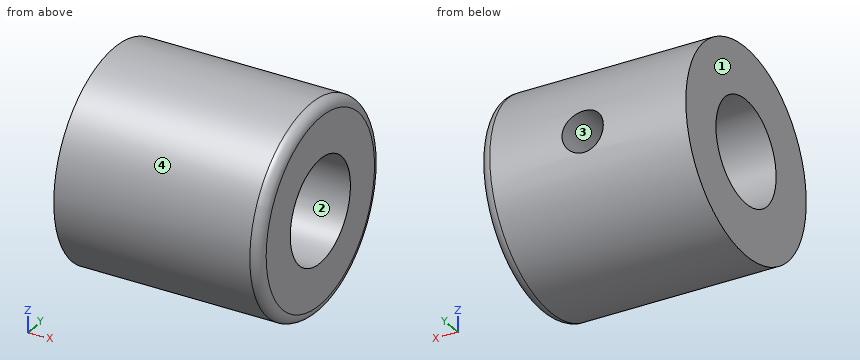
Autodesk Inventor part; units mm, degrees
ref_plane "YZ Plane" through (0, 0, 0) normal (1, 0, 0) x (0, 1, 0)
ref_plane "XZ Plane" through (0, 0, 0) normal (0, 1, 0) x (-1, 0, 0)
ref_plane "XY Plane" through (0, 0, 0) normal (0, 0, 1) x (1, 0, 0)
sketch "Sketch1" plane through (0, 0, 0) normal (1, 0, 0) x (0, 1, 0)
  circle A0 centre (0, 0) radius 2.5
  circle A1 centre (0, 0) radius 5
  dimension "d0" = 5
  dimension "d1" = 10
extrude "Extrusion1" add sketch "Sketch1" along normal blind 10
sketch "Sketch2" plane through (0, 0, 0) normal (0, 1, 0) x (-1, 0, 0)
  line L0 (0, 0) -> (-5, 0)
  circle A0 centre (-5, 0) radius 1
  dimension "d4" = 5
  dimension "d5" = 2
extrude "Extrusion2" cut sketch "Sketch2" along normal blind 10
thread "Thread1"
fillet "Fillet1" radius 0.5 1 edges at (10, -5, 0)
properties part number "wormgear_worm_axes_holder" material "Aluminum 6061"
Model file for the job. Use its own axes, mm. Face numbers are marked on the shaded views. Give positions to 0.01 mm unless a question says otherwise; leave off trailing zeros. Loops run counter-clockwise (first coordinate to the right, second up) from the corner with the lowest first, then second, coordinate; pieces in that order, holes last.
Item 1: Slice it at B-B (z = 0). Write the cut outline in (x, y), plus the area to 3 significant figures.
Check values:
outline: (0, -5) - (9.5, -5) arc R0.5 ccw to (10, -4.5) - (10, -2.5) - (0, -2.5) - close; (0, 2.5) - (4, 2.5) - (4, 5) - (0, 5) - close; (6, 2.5) - (10, 2.5) - (10, 4.5) arc R0.5 ccw to (9.5, 5) - (6, 5) - close
area: 44.9 mm2
Item 2: Slice it at C-C (x = 7.25). Write the cut outline in (y, z), plus the area to 3 significant figures.
Check values:
outline: circle Ø10 at (0, 0); hole circle Ø5 at (0, 0)
area: 58.9 mm2
Item 3: Mould opens along Z. For the marked faces 1, 2, 3 and 4 say: +Z half, -Z half, draft (parallel to the pull), parting line (faces both ways), or undercut.
Check values:
face 1: draft
face 2: undercut
face 3: undercut
face 4: parting line
Item 4: Drop a flat-ended pin along its axis: P1, Ø1.5, axis at x = 4, z = 1, coming from the +Y side. Give the stop position or say it passes through.
Check values:
P1: stops at y = 4.99
Item 5: Drill centre lines: line 1 along X through (y, z) = (2.9, 0); line 2 along Z through (x, y) = (4, 0); line 3 along Z through (x, y) = (5, 4.05). Where is each one in solid material? Low to high.
Check values:
line 1: x = 0 to 4, 6 to 10
line 2: z = -5 to -2.5, 2.5 to 5
line 3: z = -2.93 to -1, 1 to 2.93
Item 6: Slice it at D-D (x = 4.5). Write the cut outline in (y, z), plus the area to 3 significant figures.
Check values:
outline: (2.35, -0.87) arc R2.5 cw (long way) to (2.35, 0.87) - (4.92, 0.87) arc R5 ccw (long way) to (4.92, -0.87) - close
area: 54.5 mm2
Item 7: Slice it at A-A (y = 0). Write the cut outline in (x, z), plus the area to 3 significant figures.
Check values:
outline: (0, -5) - (9.5, -5) arc R0.5 ccw to (10, -4.5) - (10, -2.5) - (0, -2.5) - close; (0, 2.5) - (10, 2.5) - (10, 4.5) arc R0.5 ccw to (9.5, 5) - (0, 5) - close
area: 49.9 mm2
